CAD build for the part. Positions are in the model's coordinates, mm. Face numbers are marked on the shaded views. Round coordinates to 2 decimals unless told otherwise and drop trailing zeros. Loops run counter-clockwise (first coordinate to the right, second up) from the corner with the lowest first, then second, coordinate; pieces in that order, holes last. Notation, with made-up numbers: M -24,37.25 L 25,37.25 A30 ccw 25,74.25 Z; hole C 33.5,2 d1. An arc over 180 degrees is marked long. One line per item, written item: value. Start each with the question number.
from build123d import *

# Parameters (mm, degrees)
SKETCH1_R          = 1.375
SKETCH1_R_2        = 5
EXTRUDE1_DEPTH     = 3
SKETCH2_R          = 1.6
CUT_EXTRUDE1_DEPTH = 3
SKETCH3_R          = 1.6
EXTRUDE2_DEPTH     = 2
EXTRUDE3_DEPTH     = 2
SKETCH5_R          = 1.35
CUT_EXTRUDE2_DEPTH = 5
CHAMFER1_SIZE      = 1


with BuildPart() as part:
    # Sketch1 → Extrude1 (new body)
    with BuildSketch(Plane.XY):
        with BuildLine():
            Line((9, 72), (-20.691500947, 72))
            ThreePointArc((-20.691500947, 72), (-25.583940659, 68.031520074), (-30.476380371, 72))
            Line((-30.476380371, 72), (-61.523619629, 72))
            ThreePointArc((-61.523619629, 72), (-66.416059341, 68.031520074), (-71.308499053, 72))
            Line((-71.308499053, 72), (-101, 72))
            Line((-101, 72), (-111, 62))
            Line((-111, 62), (-111, -17))
            Line((-111, -17), (-101, -27))
            Line((-101, -27), (9, -27))
            Line((9, -27), (19, -17))
            Line((19, -17), (19, 62))
            Line((19, 62), (9, 72))
        make_face()
        with Locations((-86, 0)):
            Circle(SKETCH1_R, mode=Mode.SUBTRACT)
        with Locations((-86, 58)):
            Circle(SKETCH1_R, mode=Mode.SUBTRACT)
        Circle(SKETCH1_R, mode=Mode.SUBTRACT)
        with Locations((0, 58)):
            Circle(SKETCH1_R, mode=Mode.SUBTRACT)
        with Locations((-7.462680425, -16.037319575)):
            Circle(SKETCH1_R_2, mode=Mode.SUBTRACT)
        with Locations((-84.537319575, -16.037319575)):
            Circle(SKETCH1_R_2, mode=Mode.SUBTRACT)
    extrude(amount=EXTRUDE1_DEPTH)

    # Sketch2 → Cut-Extrude1 (cut)
    with BuildSketch(Plane(origin=(0, 0, 0), x_dir=(-1, 0, 0), z_dir=(0, 0, -1))):
        with Locations((-9, 52)):
            Circle(SKETCH2_R)
        with Locations((-9, -7)):
            Circle(SKETCH2_R)
        with Locations((101, 52)):
            Circle(SKETCH2_R)
        with Locations((101, -7)):
            Circle(SKETCH2_R)
        with BuildLine():
            Line((13, 60), (74, 60))
            ThreePointArc((74, 60), (77.535533906, 58.535533906), (79, 55))
            Line((79, 55), (79, 2))
            ThreePointArc((79, 2), (77.535533906, -1.535533906), (74, -3))
            Line((74, -3), (13, -3))
            ThreePointArc((13, -3), (9.464466094, -1.535533906), (8, 2))
            Line((8, 2), (8, 55))
            ThreePointArc((8, 55), (9.464466094, 58.535533906), (13, 60))
        make_face()
    extrude(amount=-CUT_EXTRUDE1_DEPTH, mode=Mode.SUBTRACT)

    # Sketch3 → Extrude2 (add)
    # profile 1 of 2: a face of its own
    with BuildSketch(Plane.XY.offset(3)):
        with BuildLine():
            Line((4, -1.068897687), (4, -7))
            ThreePointArc((4, -7), (9, -12), (14, -7))
            Line((14, -7), (14, 52))
            ThreePointArc((14, 52), (9, 57), (4, 52))
            Line((4, 52), (4, 2.241917312))
            ThreePointArc((4, 2.241917312), (4.498075539, 0.586509812), (4, -1.068897687))
        make_face()
        with Locations(Location((9, -7, 0), (0, 0, 180))):
            Circle(SKETCH3_R, mode=Mode.SUBTRACT)
        with Locations(Location((9, 52, 0), (0, 0, 180))):
            Circle(SKETCH3_R, mode=Mode.SUBTRACT)
    # profile 2 of 2: a face of its own
    with BuildSketch(Plane.XY.offset(3)):
        with BuildLine():
            Line((-96, 52), (-96, -7))
            ThreePointArc((-96, -7), (-101, -12), (-106, -7))
            Line((-106, -7), (-106, 52))
            ThreePointArc((-106, 52), (-101, 57), (-96, 52))
        make_face()
        with Locations(Location((-101, -7, 0), (0, 0, 180))):
            Circle(SKETCH3_R, mode=Mode.SUBTRACT)
        with Locations(Location((-101, 52, 0), (0, 0, 180))):
            Circle(SKETCH3_R, mode=Mode.SUBTRACT)
    extrude(amount=EXTRUDE2_DEPTH)

    # Sketch4 → Extrude3 (add)
    with BuildSketch(Plane.XY.offset(3)):
        with BuildLine():
            Line((-11, -10), (-81, -10))
            ThreePointArc((-81, -10), (-84, -7), (-81, -4))
            Line((-81, -4), (-11, -4))
            ThreePointArc((-11, -4), (-8, -7), (-11, -10))
        make_face()
    extrude(amount=EXTRUDE3_DEPTH)

    # Sketch5 → Cut-Extrude2 (cut)
    with BuildSketch(Plane(origin=(0, 0, 0), x_dir=(-1, 0, 0), z_dir=(0, 0, -1))):
        with Locations((-7, 64)):
            Circle(SKETCH5_R)
        with Locations((99, 64)):
            Circle(SKETCH5_R)
        with Locations((99, -19)):
            Circle(SKETCH5_R)
        with Locations((-7, -19)):
            Circle(SKETCH5_R)
    extrude(amount=-CUT_EXTRUDE2_DEPTH, mode=Mode.SUBTRACT)

    # Chamfer1
    chamfer1_edges = [part.edges().sort_by_distance(p)[0] for p in [
        (-87.375, 0, 3),
        (-87.375, 58, 3),
        (-1.375, 0, 3),
        (-1.375, 58, 3),
    ]]
    chamfer(chamfer1_edges, length=CHAMFER1_SIZE)


solid = part.part
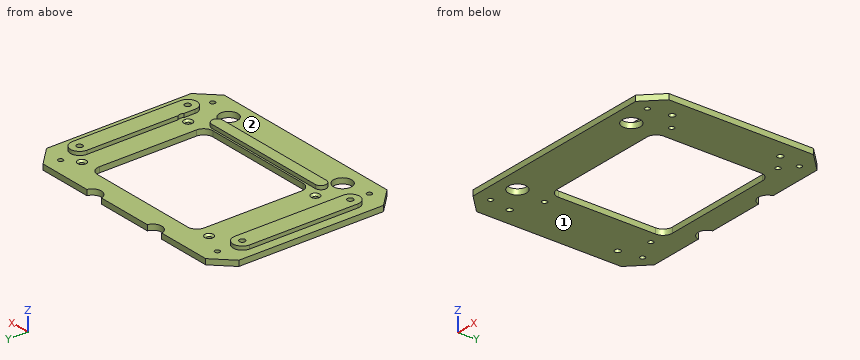
(1) Probe L1, parallel to Y at x = -101, z = 2; L2, parallel to Y at x = -101, z = 4.25; L3, parallel to X at y = 32, z = 0.5. List the from-to ranges inside material, lowest first.
(2) Mould opens along X. For the marked faces 1 and 2 say: pulls with the +X half, pulls with the -X half, needs draft (parallel to the pull), parting line crosses it, or undercut.
(3) Slice it at D-D, the plane y = -19. List the corners of the cut face in (x, z), and give its area (3 significant figures).
(4) Slice it at B-B, the plane y = 12.5. List the corners of the cut face in (x, z).
(5) Slice it at C-C, the plane x = -68.5. List the corners of the cut face in (y, z).
(6) Slice it at A-A, the plane x = 0. List the corners of the cut face in (y, z) (3 decimals), and give its area (4 significant figures).
(7) Flat gauge pins, fed straight in: P1, Ø1.9, axis at x = -101, y = -7, coming from the -Z side; P2, Ø10, axis at x = -5.5, y = 7, coming from the +Z side; P3, Ø1, axis at y = -5, z = 4.5, coming from the -X side; P4, Ø1.6, axis at x = -38, z = 4, coming from the -Y side. Where does each tip first touch, or does it go through?
Check result:
1. L1: y = -27 to -8.6, -5.4 to 50.4, 53.6 to 72
1. L2: y = -12 to -8.6, -5.4 to 50.4, 53.6 to 57
1. L3: x = -111 to -79, -8 to 19
2. face 1: needs draft
2. face 2: undercut
3. outline: M -109,0 L -100.35,0 L -100.35,3 L -109,3 Z; M -97.65,0 L -88.57,0 L -88.57,3 L -97.65,3 Z; M -80.51,0 L -11.49,0 L -11.49,3 L -80.51,3 Z; M -3.43,0 L 5.65,0 L 5.65,3 L -3.43,3 Z; M 8.35,0 L 17,0 L 17,3 L 8.35,3 Z
3. area: 313 mm^2
4. outline: M -111,0 L -79,0 L -79,3 L -96,3 L -96,5 L -106,5 L -106,3 L -111,3 Z; M -8,0 L 19,0 L 19,3 L 14,3 L 14,5 L 4,5 L 4,3 L -8,3 Z
5. outline: M -27,0 L -3,0 L -3,3 L -4,3 L -4,5 L -10,5 L -10,3 L -27,3 Z; M 60,0 L 68.49,0 L 68.49,3 L 60,3 Z
6. outline: M -27,0 L -1.375,0 L -1.375,2 L -2.375,3 L -27,3 Z; M 1.375,0 L 56.625,0 L 56.625,2 L 55.625,3 L 2.375,3 L 1.375,2 Z; M 59.375,0 L 72,0 L 72,3 L 60.375,3 L 59.375,2 Z
6. area: 278.5 mm^2
7. P1: passes through
7. P2: stops at z = 3
7. P3: stops at x = -106
7. P4: stops at y = -10
